The model under review builds one solid part; all positions refer to its coordinate system, in mm. Face numbers are marked on the shaded views. A direction names the side the tool comes from. Round coordinates to 2 decimals unless told otherwise and drop trailing zeros. Order: outer loops, then holes, each group sorted by start corner. A loop starts at its lowest first (then second) coordinate and runs counter-clockwise, first axis right, second up. Notation, with made-up numbers: M 35,79.5 L 47,79.5 A14 cw 47,96.5 Z; hole C 76.25,-14 d9. An arc over 180 degrees is marked long. Answer as a JSON object with one key per item and string values. Group by question number.
1. Machinability: for the marked faces 1, 2 and 3, which of the approach directions +Z, -Z, +X, -X, +Y, -Y give a long, thin tool a straight path to every point of the face, cutting with its end or side? Answer none if there is none.
2. Mouldability with a two-part tool opening along X and no side actions: class the marked faces 4, 5, 6 and 7 as released by +X, released by -X, zero draft, split by the parting line, or undercut.
3. Add section A-A on x = 30. State the section outline as (y, z) points.
4. Clearance check with flat-ended pins moving along their axes: P1, Ø1.5, axis at x = 17, y = -13, coming from the +Z side; P2, Ø1, axis at y = 0.5, z = 7, coming from the +X side; P3, Ø5, axis at x = 30, z = 5, coming from the +Y side. State where each tip first meets the part, or that it passes through.
5. Add section B-B on y = -8.75. State the section outline as (x, z) points, and give its area (3 significant figures).
6. To check wall thickness, follow probe 1 along Y at (x, z) = (28.75, 2); probe 2 along Z at (x, y) = (22, -4.5); probe 3 along Y at (x, z) = (14.75, 2.5). State the ranges of each line that lie inside material, in increasing order. Write a range as [from, to].
7. Add section C-C on y = -5.5. State the section outline as (x, z) points, and give its area (3 significant figures).
```python
from build123d import *

# Parameters (mm, degrees)
PAD_DEPTH           = 3
HOLE_D              = 3.2
HOLE_CSINK_D        = 6
HOLE_CSINK_ANGLE    = 90
SKETCH002_W         = 5
SKETCH002_H         = 3
SKETCH003_W         = 10.1
SKETCH003_H         = 10
SKETCH004_W         = 8
SKETCH004_H         = 3
PAD001_DEPTH        = 10
FILLET_R            = 1
POCKET_DEPTH        = 25.359393
HOLE001_D           = 3.2
HOLE001_CSINK_D     = 6
HOLE001_CSINK_ANGLE = 90
POCKET001_DEPTH     = 2


with BuildPart() as part:
    # Sketch → Pad (new body)
    with BuildSketch(Plane.XY):
        with BuildLine():
            ThreePointArc((10.912011, -11.701625), (14.672971, -6.379962), (16, 0))
            Line((16, 0), (16, 5))
            Line((26, 5), (16, 5))
            Line((26, 5), (26, 0))
            ThreePointArc((17.731994, -19.015162), (23.843572, -10.367453), (26, 0))
            ThreePointArc((10.912011, -11.701625), (10.665234, -18.768385), (17.731994, -19.015162))
        make_face()
    extrude(amount=PAD_DEPTH)

    # Hole (through all)
    with Locations(Plane.XY.offset(3)):
        with Locations((14.322002, -15.358393)):
            CounterSinkHole(HOLE_D / 2, HOLE_CSINK_D / 2, counter_sink_angle=HOLE_CSINK_ANGLE)

    # Sketch002 (on Face6 of Hole) → AdditiveLoft section 0
    with BuildSketch(Plane(origin=(16, 0, 0), x_dir=(0, -1, 0), z_dir=(-1, 0, 0))):
        with Locations((-2.5, 1.5)):
            Rectangle(SKETCH002_W, SKETCH002_H)
    # Sketch003 (on Face7 of Hole) → AdditiveLoft section 1
    with BuildSketch(Plane.YZ.offset(26)):
        with Locations((-0.05, 5)):
            Rectangle(SKETCH003_W, SKETCH003_H)
    loft()

    # Sketch004 → Pad001 (join)
    with BuildSketch(Plane.XY):
        with Locations((30, 3.5)):
            Rectangle(SKETCH004_W, SKETCH004_H)
        with Locations((30, -3.6)):
            Rectangle(SKETCH004_W, SKETCH004_H)
    extrude(amount=PAD001_DEPTH)

    # Fillet
    fillet_edges = [part.edges().sort_by_distance(p)[0] for p in [
        (26, 2, 5),
        (26, -2.1, 5),
    ]]
    fillet(fillet_edges, radius=FILLET_R)

    # Sketch005 (on Face14 of Fillet) → Pocket (cut, through all)
    with BuildSketch(Plane(origin=(0, 5, 0), x_dir=(-1, 0, 0), z_dir=(0, 1, 0))):
        with BuildLine():
            Line((-34, 10), (-28.1, 10))
            ThreePointArc((-28.1, 10), (-32.27193, 8.27193), (-34, 4.1))
            Line((-34, 10), (-34, 4.1))
        make_face()
        with BuildLine():
            Line((-34, 0), (-34, 5.9))
            ThreePointArc((-34, 5.9), (-32.27193, 1.72807), (-28.1, 0))
            Line((-34, 0), (-28.1, 0))
        make_face()
    extrude(amount=-POCKET_DEPTH, mode=Mode.SUBTRACT)

    # Hole001 (through all)
    with Locations(Plane(origin=(0, 5, 0), x_dir=(-1, 0, 0), z_dir=(0, 1, 0))):
        with Locations((-30, 5)):
            CounterSinkHole(HOLE001_D / 2, HOLE001_CSINK_D / 2, counter_sink_angle=HOLE001_CSINK_ANGLE)

    # Sketch007 (on Face17 of Hole001) → Pocket001 (cut)
    with BuildSketch(Plane.XZ.offset(5.1)):
        Polygon((33.348632, 5), (31.674316, 7.9), (28.325684, 7.9), (26.651368, 5), (28.325684, 2.1), (31.674316, 2.1), align=None)
    extrude(amount=-POCKET001_DEPTH, mode=Mode.SUBTRACT)


solid = part.part
```
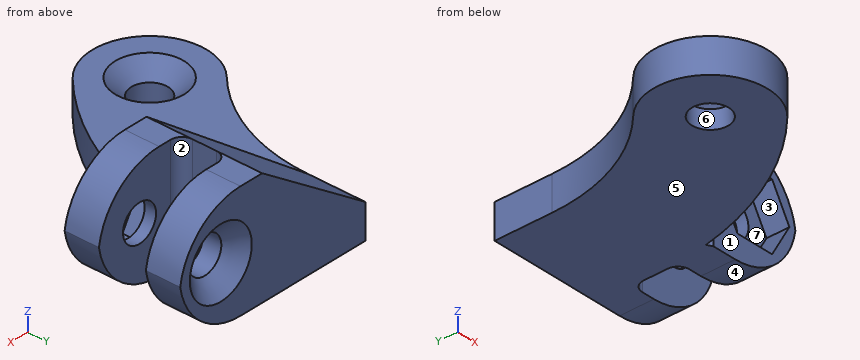
Recorded:
{
 "1": {"face 1": "+Z, -Z, +X, -Y", "face 2": "+Z, -Z, +X", "face 3": "-Y"},
 "2": {"face 4": "released by +X", "face 5": "zero draft", "face 6": "undercut", "face 7": "undercut"},
 "3": {"outline": "M -5.1,0.31 L -2.1,0.31 L -2.1,3.4 L -3.1,3.4 L -3.1,2.1 L -5.1,2.1 Z; M -5.1,7.9 L -3.1,7.9 L -3.1,6.6 L -2.1,6.6 L -2.1,9.69 L -5.1,9.69 Z; M 2,0.31 L 5,0.31 L 5,2 L 3.6,3.4 L 2,3.4 Z; M 2,6.6 L 3.6,6.6 L 5,8 L 5,9.69 L 2,9.69 Z"},
 "4": {"P1": "stops at z = 3", "P2": "stops at x = 26", "P3": "stops at y = 4.5"},
 "5": {"outline": "M 13.4,0 L 24.48,0 L 24.48,3 L 13.4,3 Z", "area": "33.3 mm²"},
 "6": {"probe 1": "y = [-5.1, -2.1], [2, 5]", "probe 2": "z = [0, 3]", "probe 3": "y = [-20.34, -17.82], [-12.9, -6.2]"},
 "7": {"outline": "M 15.02,0 L 25.41,0 L 25.41,3 L 15.02,3 Z", "area": "31.2 mm²"}
}
